Read the model definition and answer for the solid it produces. Units are mm, in the model's axes. A direction names the side the tool comes from. Give positions to 0.01 mm unless a question says otherwise; leave off trailing zeros. Order: outer loops, then holes, each group sorted by start corner. A loop starts at its lowest first (then second) coordinate and runs counter-clockwise, first axis right, second up. Notation, with made-up numbers: M 81,39.5 L 109,39.5 A12 cw 109,47.5 Z; hole C 33,82.5 d7. An arc over 180 degrees is marked long. Write item = value, one per line. Start each with the question number.
from build123d import *

# Parameters (mm, degrees)
F0_W      = 38.1
F0_H      = 38.1
F1_DEPTH  = 7.62
F2_W      = 1.8288
F2_H      = 13.97
F3_DEPTH  = 38.101
F4_W      = 13.97
F4_H      = 1.8288
F5_DEPTH  = 38.101
F6_W      = 17.78
F6_H      = 17.78
F7_DEPTH  = 7.621
F8_R      = 2.54
F9_R      = 1.7
F10_DEPTH = 7.621
F11_R     = 1.27


with BuildPart() as f1:
    # F0 (on Front) → F1 (new body)
    with BuildSketch(Plane.XZ):
        with Locations((19.05, 19.05)):
            Rectangle(F0_W, F0_H)
    extrude(amount=F1_DEPTH)

    # F2 (on face) → F3 (cut, through all)
    with BuildSketch(Plane.YZ.offset(38.1)):
        with Locations((-3.81, 6.985)):
            Rectangle(F2_W, F2_H)
    extrude(amount=-F3_DEPTH, mode=Mode.SUBTRACT)

    # F4 (on face) → F5 (cut, through all)
    with BuildSketch(Plane.XY.offset(38.1)):
        with Locations((6.985, -3.81)):
            Rectangle(F4_W, F4_H)
    extrude(amount=-F5_DEPTH, mode=Mode.SUBTRACT)

    # F6 (on face) → F7 (cut, through all)
    with BuildSketch(Plane(origin=(0, 0, 0), x_dir=(-1, 0, 0), z_dir=(0, 1, 0))):
        with Locations((-29.21, 29.21)):
            Rectangle(F6_W, F6_H)
    extrude(amount=-F7_DEPTH, mode=Mode.SUBTRACT)

    # F8
    f8_edges = [f1.edges().sort_by_distance(p)[0] for p in [
        (13.97, -3.81, 13.97),
    ]]
    fillet(f8_edges, radius=F8_R)

    # F9 (on face) → F10 (cut, through all)
    with BuildSketch(Plane.XZ.offset(7.62)):
        with Locations((6.985, 25.4)):
            Circle(F9_R)
        with BuildLine():
            ThreePointArc((23.7, 6.985), (24.197918472, 5.782918472), (25.4, 5.285))
            Line((25.4, 5.285), (25.4, 6.985))
            Line((25.4, 6.985), (23.7, 6.985))
        make_face()
        with BuildLine():
            Line((25.4, 6.985), (25.4, 5.285))
            ThreePointArc((25.4, 5.285), (26.602081528, 5.782918472), (27.1, 6.985))
            ThreePointArc((27.1, 6.985), (25.4, 8.685), (23.7, 6.985))
            Line((23.7, 6.985), (25.4, 6.985))
        make_face()
    extrude(amount=-F10_DEPTH, mode=Mode.SUBTRACT)

    # F11
    f11_edges = [f1.edges().sort_by_distance(p)[0] for p in [
        (10.16, 0, 38.1),
        (10.16, -7.62, 38.1),
        (20.32, -3.81, 38.1),
        (20.32, 0, 29.21),
        (20.32, -7.62, 29.21),
        (20.32, -3.81, 20.32),
        (38.1, -3.81, 20.32),
        (29.21, 0, 20.32),
        (29.21, -7.62, 20.32),
        (38.1, 0, 10.16),
        (38.1, -7.62, 10.16),
    ]]
    fillet(f11_edges, radius=F11_R)


solid = f1.part
1) For faces 1 (the face through (38.1, -2.6, 9.4)), 2 (the face through (29.103, -0.362, 19.938)), 3 (the face through (10, -4.724, 15)), determine the directions among +Z, -Z, +X, -X, +Y, -Y from which every point of the face is accessible in a straight line to the end or side of a thin tool.
2) Find the intervals of material crossed by probe 1 along Y at (x, z) = (4, 7); probe 2 along Z at (x, y) = (36, -3); probe 3 along Z at (x, y) = (17, -3.25), in increasing order. Write a range as [from, to].
3) Find section C-C on x = 4.5. Determine the outline of the cut face in (y, z).
4) Find section A-A on z = 12.5. Determine the outline of the cut face in (x, y).
5) For a pull along X with two mould halves and no side action, classify faces 4 (the face through (19, -6, 0)), 5 (the face through (20.702, -3.846, 20.682)), 6 (the face through (6.62, -6.19, 23.74)), 7 (the face through (13.97, -4, 27)) as pulls with the +X half, pulls with the -X half, needs draft (parallel to the pull), parting line crosses it, or undercut.
6) Find section B-B on y = -5.25. Determine the outline of the cut face in (x, z) (3 decimals), plus the area to 3 significant figures.
7) Each of these flat-tipped pins is pushed along its axis until it touches: P1, Ø1.5, axis at y = -3, z = 30.5, coming from the +X side; P2, Ø2, axis at x = 33.5, y = -4.5, coming from the +Z side; P3, Ø0.5, axis at y = -3.5, z = 27.5, coming from the -X side. Where does it stop, or does it pass through?
8) Find section D-D on z = 29.5. Determine the outline of the cut face in (x, y), plus the area to 3 significant figures.
Numbers:
q1.face_1 = +Z, -Z, +X, +Y, -Y
q1.face_2 = +Z, +X, +Y
q1.face_3 = -Z, -X
q2.probe_1 = [-7.62, -4.72], [-2.9, 0]
q2.probe_2 = [13.97, 20.32]
q2.probe_3 = [13.97, 38.1]
q3.outline = M -7.62,0 L -4.72,0 L -4.72,38.1 L -6.35,38.1 A1.27 ccw -7.62,36.83 Z; M -2.9,0 L 0,0 L 0,36.83 A1.27 ccw -1.27,38.1 L -2.9,38.1 Z
q4.outline = M 0,-7.62 L 36.83,-7.62 A1.27 ccw 38.1,-6.35 L 38.1,-4.72 L 0,-4.72 Z; M 0,-2.9 L 38.1,-2.9 L 38.1,-1.27 A1.27 ccw 36.83,0 L 0,0 Z
q5.face_4 = needs draft
q5.face_5 = pulls with the +X half
q5.face_6 = undercut
q5.face_7 = pulls with the -X half
q6.outline = M 0,0 L 38.1,0 L 38.1,19.05 A1.27 ccw 36.83,20.32 L 21.59,20.32 A1.27 cw 20.32,21.59 L 20.32,36.83 A1.27 ccw 19.05,38.1 L 0,38.1 Z; hole C 6.985,25.4 d3.4; hole C 25.4,6.985 d3.4
q6.area = 1,120 mm2
q7.P1 = 20.32
q7.P2 = 20.32
q7.P3 = 13.97
q8.outline = M 0,-7.62 L 19.05,-7.62 A1.27 ccw 20.32,-6.35 L 20.32,-1.27 A1.27 ccw 19.05,0 L 0,0 L 0,-2.9 L 13.97,-2.9 L 13.97,-4.72 L 0,-4.72 Z
q8.area = 129 mm2
